Design review of the part shown in the three views and the two pictorial views. Dimensions are in mm from the part's minimum x, y and z. A direction names the side the tool comes from. Coordinates: 2 decimals unless noted, no trailing zeros. Loops run counter-clockwise (first coordinate to the right, second up) from the corner with the lowest first, then second, coordinate; pieces in that order, holes last. Notation, with made-up numbers: (46.5, 1.5) -> (95.5, 1.5) arc R20 ccw to (95.5, 13.5) -> close; hole circle Ø6 at (67.5, 20.5). An arc over 180 degrees is marked (long way). Answer in a Markdown table with one row per item.
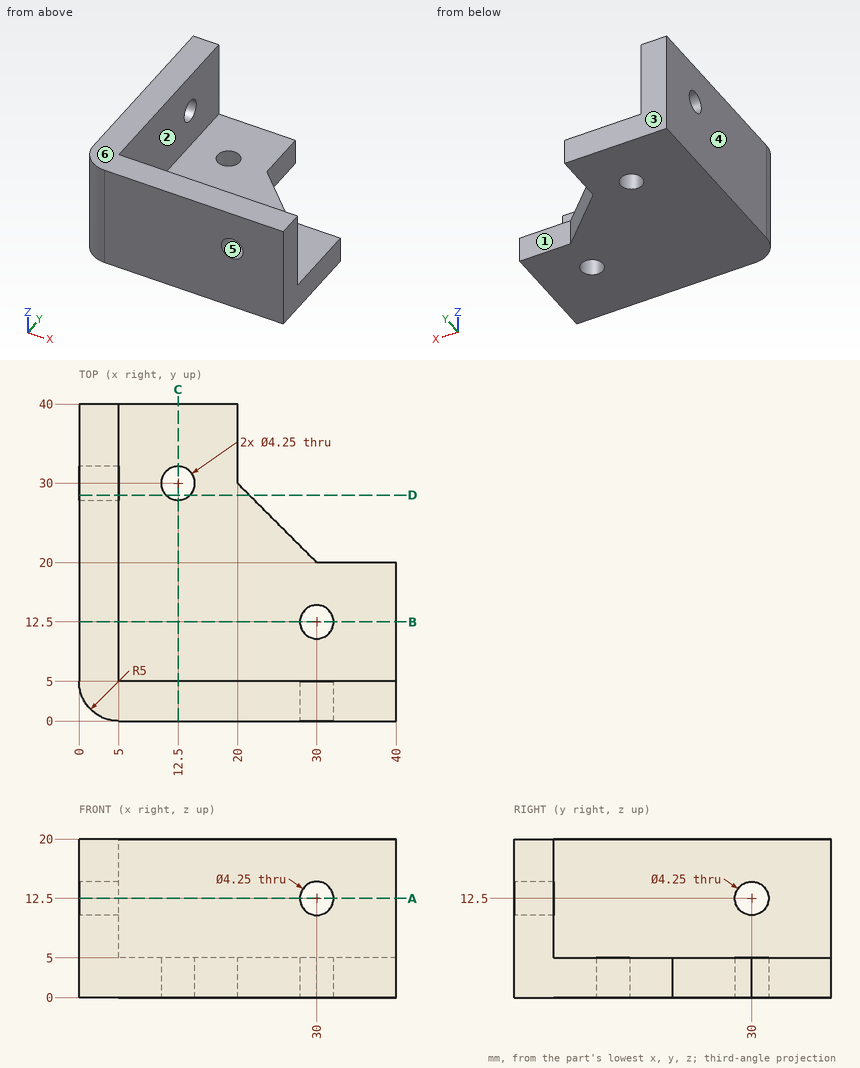
(1) Tool access review of the marked faces 1, 2 and 3: name each direction out of +Z, -Z, +X, -X, +Y, -Y from which nothing blocks a thin tool from reaching the whole face with its end or side.
Evaluation:
| item | result |
|---|---|
| face 1 | +Z, -Z, +X, +Y |
| face 2 | +Z, +X, +Y |
| face 3 | +Z, -Z, +X, -X, +Y |
(2) Draft analysis for pull direction Z (two halves, no side actions). For the marked faces 4, 5 and 6, state which applies: pulls with the +Z half, pulls with the -Z half, needs draft (parallel to the pull), parting line crosses it, or undercut.
Evaluation:
| item | result |
|---|---|
| face 4 | needs draft |
| face 5 | undercut |
| face 6 | pulls with the +Z half |
(3) To check wall thickness, follow probe 1 along Y at (x, z) = (30, 3.6) (3 decimals); probe 2 along Z at (x, y) = (14, 18). State the ranges of each line that lie inside material, in increasing order.
Evaluation:
| item | result |
|---|---|
| probe 1 | y = 0 to 10.375, 14.625 to 20 |
| probe 2 | z = 0 to 5 |
(4) Take a section at A-A on z = 12.5. Give the boundary of the cut face in (x, y) (3 decimals).
Evaluation:
| item | result |
|---|---|
| outline | (0, 5) arc R5 ccw to (5, 0) -> (27.875, 0) -> (27.875, 5) -> (5, 5) -> (5, 27.875) -> (0, 27.875) -> close; (0, 32.125) -> (5, 32.125) -> (5, 40) -> (0, 40) -> close; (32.125, 0) -> (40, 0) -> (40, 5) -> (32.125, 5) -> close |
(5) Take a section at D-D on y = 28.5. Give the boundary of the cut face in (x, z), and give its area (3 significant figures).
Evaluation:
| item | result |
|---|---|
| outline | (0, 0) -> (10.99, 0) -> (10.99, 5) -> (5, 5) -> (5, 10.99) -> (0, 10.99) -> close; (0, 14.01) -> (5, 14.01) -> (5, 20) -> (0, 20) -> close; (14.01, 0) -> (21.5, 0) -> (21.5, 5) -> (14.01, 5) -> close |
| area | 152 mm² |
(6) Take a section at B-B on y = 12.5. Give the boundary of the cut face in (x, z) (3 decimals), and give its area (3 significant figures).
Evaluation:
| item | result |
|---|---|
| outline | (0, 0) -> (27.875, 0) -> (27.875, 5) -> (5, 5) -> (5, 20) -> (0, 20) -> close; (32.125, 0) -> (40, 0) -> (40, 5) -> (32.125, 5) -> close |
| area | 254 mm² |
(7) For pin 1 (4 mm diameter, centred on y = 33, z = 2, fed in from +X); pin 2 (6 mm diameter, centred on x = 29, z = 16.5, fed in from +Y); pin 3 (5.5 mm diameter, centred on x = 35.5, z = 2.5, fed in from +Y), all flat-tipped, find the tip position at first contact; note any pin that passes through.
Evaluation:
| item | result |
|---|---|
| pin 1 | stops at x = 20 |
| pin 2 | stops at y = 5 |
| pin 3 | stops at y = 20 |
